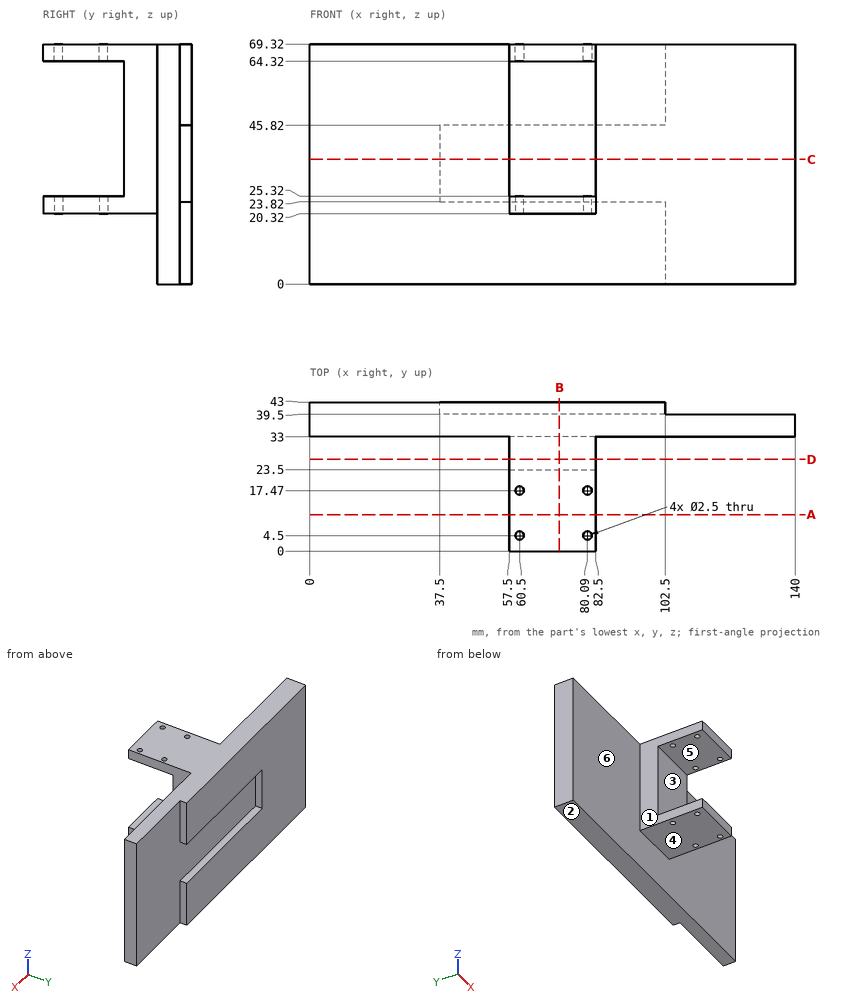
Drawing for the job (mm, zero at the part's lowest x, y, z). A direction names the side the tool comes from. Give positions to 0.01 mm unless a question says otherwise; leave off trailing zeros. Write each loop counter-clockwise with the first axis right and the second up, starting at its lowest first coordinate (ties: lowest second). Pieces come first, ordered by that corner, then holes. Notation, with made-up numbers: M 34,85.25 L 47,85.25 A18 cw 47,110.25 Z; hole C 7.25,37 d2. An arc over 180 degrees is marked long. Return JSON: item names as keys, results as strings. Group by question number.
(1) Band-saw the part on B-B (x = 72). Give the cut face in (y, z), and give its area (3 significant figures).
(2) Band-saw the part on D-D (y = 26.5). Give the cut face in (x, z).
(3) Band-saw the part on A-A (y = 10.5). Give the cut face in (x, z), and give its area (3 significant figures).
(4) 3-axis set-ups, long thin cutter, end or side, ignore diameter. For the marked faces 1, 2 and 3: which of +Z, -Z, +X, -X, +Y, -Y reach the whole face in a straight line?
(5) Drill centre lines: L1, parallel to Y at x = 80.09, z = 66.25; L2, parallel to X at y = 17, z = 23; L3, parallel to X at y = 4, z = 65. Where is each one in solid material? Low to high. Write a range as [from, to].
(6) Band-saw the part on C-C (z = 36). Give the cut face in (x, y).
(7) Flat gauge pins, fed straight in: pin 1 Ø3 at (x, z) = (77.5, 41.5) entering from -Y; pin 2 Ø12 at (x, y) = (64, 6.5) entering from -Z; pin 3 Ø4 at (x, z) = (101.5, 27) entering from -Y; pin 4 Ø2 at (x, y) = (60.5, 4.5) entering from +Z. Where does each tip first touch, or does it go through?
(8) Mould opens along Z. For the marked faces 4, 5 and 6 say: pulls with the +Z half, pulls with the -Z half, needs draft (parallel to the pull), parting line crosses it, or undercut.
Entries:
{
 "1": {"outline": "M 0,20.32 L 33,20.32 L 33,0 L 43,0 L 43,23.82 L 39.5,23.82 L 39.5,45.82 L 43,45.82 L 43,69.32 L 0,69.32 L 0,64.32 L 23.5,64.32 L 23.5,25.32 L 0,25.32 Z", "area": "1,320 mm^2"},
 "2": {"outline": "M 57.5,20.32 L 82.5,20.32 L 82.5,69.32 L 57.5,69.32 Z"},
 "3": {"outline": "M 57.5,20.32 L 82.5,20.32 L 82.5,25.32 L 57.5,25.32 Z; M 57.5,64.32 L 82.5,64.32 L 82.5,69.32 L 57.5,69.32 Z", "area": "250 mm^2"},
 "4": {"face 1": "+Z, -Z, -X, -Y", "face 2": "-Z, +X, -X, +Y, -Y", "face 3": "+X, -X, -Y"},
 "5": {"L1": "y = [0, 3.25], [5.75, 16.22], [18.72, 43]", "L2": "x = [57.5, 59.34], [61.66, 78.93], [81.25, 82.5]", "L3": "x = [57.5, 59.35], [61.65, 78.94], [81.24, 82.5]"},
 "6": {"outline": "M 0,33 L 57.5,33 L 57.5,23.5 L 82.5,23.5 L 82.5,33 L 140,33 L 140,39.5 L 37.5,39.5 L 37.5,43 L 0,43 Z"},
 "7": {"pin 1": "stops at y = 23.5", "pin 2": "stops at z = 20.32", "pin 3": "stops at y = 33", "pin 4": "passes through"},
 "8": {"face 4": "pulls with the -Z half", "face 5": "undercut", "face 6": "needs draft"}
}
